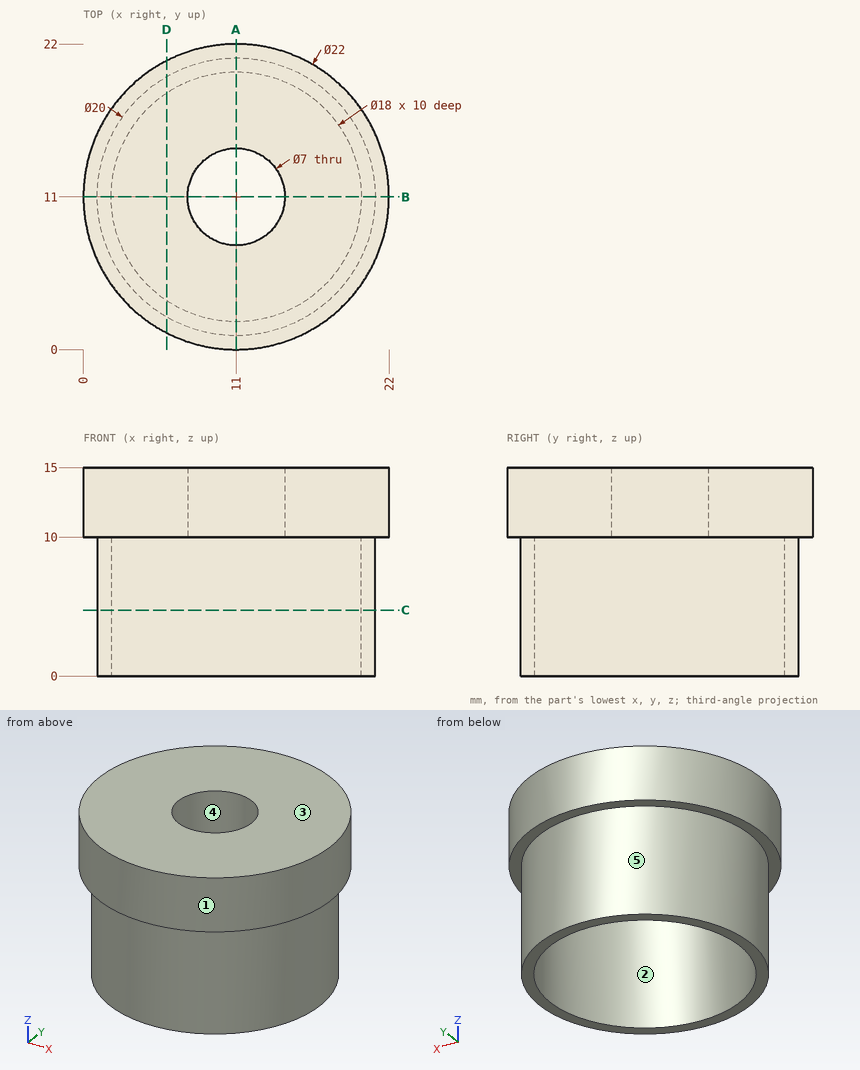
Study the drawing (mm; zero at the part's minimum x, y, z) and answer. A direction names the side the tool comes from. Coordinates: 2 decimals unless noted, no trailing zeros. Order: outer loops, then holes, each group sorted by start corner. A loop starts at its lowest first (then second) coordinate and runs counter-clockwise, first axis right, second up. Notation, with made-up numbers: M 16,32.25 L 44,32.25 A33 cw 44,64.25 Z; hole C -34,-25.75 d3. An arc over 180 degrees is marked long. Answer as a JSON object with one key per item and string values. Group by question number.
1. Straight lines are drawn through the part: line 1 (Y direction, x = 11, z = 12.1); line 2 (Y direction, x = 10.75, z = 7.5); line 3 (Z direction, x = 19, y = 4). For each, find the intervals that lie inside material, in ascending order.
2. Section A-A on x = 11 is taken. Write down the section's boundary in (y, z), then the cut area to 3 significant figures.
3. A tool of negligible diameter and unlimited length cuts with its end or side. For the marked faces 1 and 2, from which of +Z, -Z, +X, -X, +Y, -Y can it reach the whole face along a straight path? Write none if from no direction.
4. Section D-D on x = 6 is taken. Write down the section's boundary in (y, z).
5. Flat-ended cylindrical pins translate along their axes: P1, Ø4, axis at x = 18.5, z = 3, coming from the -Y side; P2, Ø6, axis at x = 5, z = 3, coming from the -Y side; P3, Ø9, axis at x = 12.5, y = 10.5, coming from the -Z side. Find the tip coordinate at first contact, or state that the pin passes through.
6. Determine the mould class of the marked faces 3, 4 and 5 for opening direction Y: released by +Y, released by -Y, zero draft, split by the parting line, or undercut.
7. Section C-C on z = 4.75 is taken. Write down the section's boundary in (x, y).
Values follow:
{
 "1": {"line 1": "0 to 7.5, 14.5 to 22", "line 2": "1 to 2, 20 to 21", "line 3": "10 to 15"},
 "2": {"outline": "M 0,10 L 1,10 L 1,0 L 2,0 L 2,10 L 7.5,10 L 7.5,15 L 0,15 Z; M 14.5,10 L 20,10 L 20,0 L 21,0 L 21,10 L 22,10 L 22,15 L 14.5,15 Z", "area": "95.0 mm2"},
 "3": {"face 1": "+Z, -Z", "face 2": "-Z"},
 "4": {"outline": "M 1.2,10 L 2.34,10 L 2.34,0 L 3.52,0 L 3.52,10 L 18.48,10 L 18.48,0 L 19.66,0 L 19.66,10 L 20.8,10 L 20.8,15 L 1.2,15 Z"},
 "5": {"P1": "y = 2.65", "P2": "y = 1.46", "P3": "z = 10"},
 "6": {"face 3": "zero draft", "face 4": "undercut", "face 5": "split by the parting line"},
 "7": {"outline": "C 11,11 d20; hole C 11,11 d18"}
}
